For this review, take the finished solid that the model builds, in its own axes (mm). Face numbers are marked on the shaded views. A direction names the side the tool comes from. Give positions to 0.01 mm unless a question says otherwise; leave off trailing zeros. Loops run counter-clockwise (first coordinate to the right, second up) from the corner with the lowest first, then second, coordinate; pieces in that order, holes last.
```python
from build123d import *

# Parameters (mm, degrees)
F0_R      = 89
F2_ANGLE  = 90
F3_R      = 141.5
F4_DEPTH  = 27
F5_R      = 141.5
F6_DEPTH  = 27
F7_R      = 9
F8_DEPTH  = 27
F9_R      = 9
F10_DEPTH = 27


with BuildPart() as f2:
    # F0 (on Front) → F2 (revolve)
    with BuildSketch(Plane.XZ):
        Circle(F0_R)
    revolve(axis=Axis((-94.423547, 0, -205), (-1, 0, 0)), revolution_arc=F2_ANGLE)

    # F3 (on face) → F4 (join)
    with BuildSketch(Plane.XZ):
        Circle(F3_R)
    extrude(amount=F4_DEPTH)

    # F5 (on face) → F6 (join)
    with BuildSketch(Plane(origin=(0, 0, -205), x_dir=(1, 0, 0), z_dir=(0, 0, -1))):
        with Locations((0, -205)):
            Circle(F5_R)
    extrude(amount=F6_DEPTH)

    # F7 (on face) → F8 (cut, through all)
    with BuildSketch(Plane(origin=(0, 0, -232), x_dir=(1, 0, 0), z_dir=(0, 0, -1))):
        with Locations((84.852814, -289.852814)):
            Circle(F7_R)
        with Locations((84.852814, -120.147186)):
            Circle(F7_R)
        with Locations((-84.852814, -120.147186)):
            Circle(F7_R)
        with Locations((-84.852814, -289.852814)):
            Circle(F7_R)
    extrude(amount=-F8_DEPTH, mode=Mode.SUBTRACT)

    # F9 (on face) → F10 (cut, through all)
    with BuildSketch(Plane.XZ.offset(27)):
        with Locations((-84.852814, 84.852814)):
            Circle(F9_R)
        with Locations((-84.852814, -84.852814)):
            Circle(F9_R)
        with Locations((84.852814, -84.852814)):
            Circle(F9_R)
        with Locations((84.852814, 84.852814)):
            Circle(F9_R)
    extrude(amount=-F10_DEPTH, mode=Mode.SUBTRACT)


solid = f2.part
```
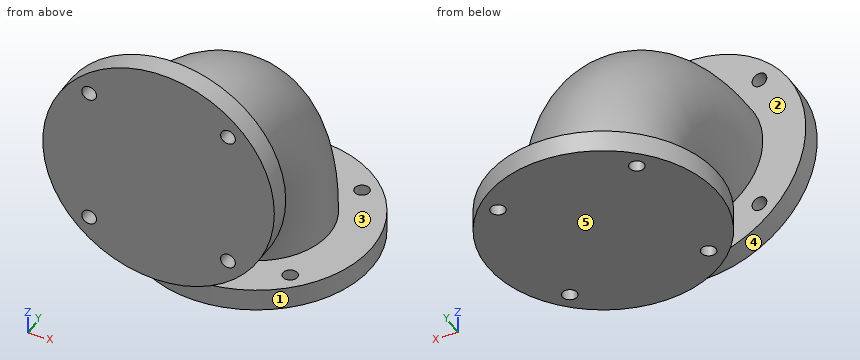
Item 1: Take a section at B-B on x = 50.5. Give the boundary of the cut face in (y, z).
Answer:
outline: (-27, -132.18) - (0, -132.18) - (0, -73.29) arc R131.71 cw to (131.71, -205) - (72.82, -205) - (72.82, -232) - (337.18, -232) - (337.18, -205) - (278.29, -205) arc R278.29 ccw to (0, 73.29) - (0, 132.18) - (-27, 132.18) - close
Item 2: The part is to be moulded in two halves that separate along Y. For the marked faces 1, 2 and 3, say which applies: released by +Y, released by -Y, zero draft, split by the parting line, or undercut.
Answer:
face 1: split by the parting line
face 2: undercut
face 3: zero draft
Item 3: For L1, parallel to Z at x = -70.5, y = 270.5; L2, parallel to Z at x = 36.5, y = 114; L3, parallel to Z at x = -32, y = 83.5, list the stretches that pass through material, from the lowest coordinate up.
Answer:
L1: z = -232 to -205
L2: z = -232 to -205, -156.65 to 57.48
L3: z = -232 to -205, -116.12 to 70.68
Item 4: Clearance check with flat-ended pins moving along their axes: pin 1 Ø1 at (y, z) = (215.5, -71.5) entering from -X; pin 2 Ø4 at (x, y) = (20, 114.5) entering from +Z; pin 3 Ø20.5 at (x, y) = (-84.85, 120.15) entering from +Z; pin 4 Ø14.5 at (x, y) = (-84.85, 289.85) entering from -Z. State where each tip first meets the part, or that it passes through.
Answer:
pin 1: stops at x = -74.95
pin 2: stops at z = 64.29
pin 3: stops at z = 19.06
pin 4: passes through
Item 5: Take a section at A-A on x = 0. Give the boundary of the cut face in (y, z).
Answer:
outline: (-27, -141.5) - (0, -141.5) - (0, -89) arc R116 cw to (116, -205) - (63.5, -205) - (63.5, -232) - (346.5, -232) - (346.5, -205) - (294, -205) arc R294 ccw to (0, 89) - (0, 141.5) - (-27, 141.5) - close
Item 6: Tool access review of the marked faces 4 and 5: name each direction out of +Z, -Z, +X, -X, +Y, -Y from which nothing blocks a thin tool from reaching the whole face with its end or side.
Answer:
face 4: -Y
face 5: -Z, +X, -X, +Y, -Y
